Source: three-view drawing plus pictorial views. Frame: mm from the lowest corner of the part. Give positions to 0.01 mm unless a question says otherwise; leave off trailing zeros. Loops run counter-clockwise (first coordinate to the right, second up) from the corner with the lowest first, then second, coordinate; pieces in that order, holes last. Notation, with made-up numbers: (52, -6.75) -> (82, -6.75) arc R15 ccw to (82, 4.25) -> close; hole circle Ø2 at (-6, 58.5). An arc over 180 degrees is marked (long way). Put each result on its own line as item: value.
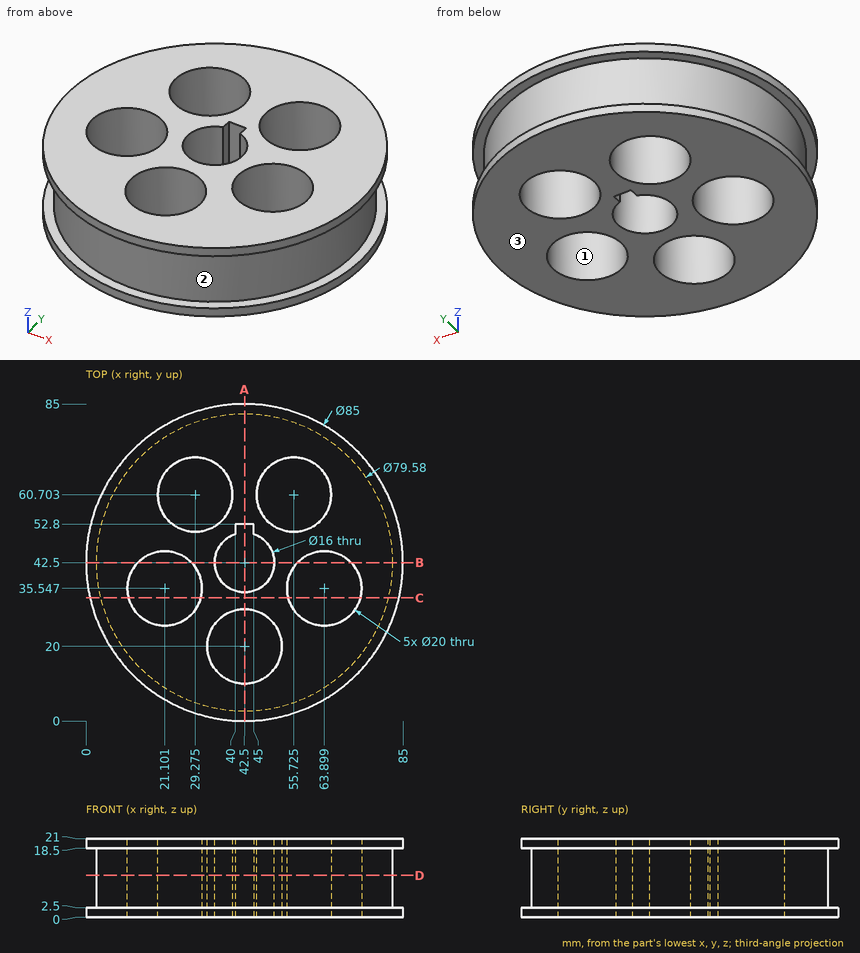
(1) Draft query along X for the marked faces 1, 2 and 3. Return one class per face: released by +X, released by -X, zero draft, split by the parting line, or undercut.
Calculated:
face 1: undercut
face 2: split by the parting line
face 3: zero draft
(2) Section C-C on y = 33. Return loops of the section in (x, z) (1 decimal).
Calculated:
outline: (1.1, 0) -> (11.4, 0) -> (11.4, 21) -> (1.1, 21) -> (1.1, 18.5) -> (3.9, 18.5) -> (3.9, 2.5) -> (1.1, 2.5) -> close; (30.8, 0) -> (54.2, 0) -> (54.2, 21) -> (30.8, 21) -> close; (73.6, 0) -> (83.9, 0) -> (83.9, 2.5) -> (81.1, 2.5) -> (81.1, 18.5) -> (83.9, 18.5) -> (83.9, 21) -> (73.6, 21) -> close
(3) First-contact query: P1, Ø1.4, axis at y = 51.5, z = 15, coming from the +X side (1 decimal); P2, Ø4, axis at y = 29, z = 6.5, coming from the +X side; P3, Ø1.5, axis at y = 56, z = 6.5, coming from the -X side. Flat tips, straight axial feed; report the tip coordinate or a pass-through.
Calculated:
P1: stops at x = 81.4
P2: stops at x = 80.59
P3: stops at x = 4.81
(4) Section D-D on z = 11.25. Return loops of the section in (x, y) (1 decimal).
Calculated:
outline: circle Ø79.6 at (42.5, 42.5); hole circle Ø20 at (21.1, 35.5); hole circle Ø20 at (29.3, 60.7); hole circle Ø20 at (42.5, 20); hole (40, 50.1) arc R8 ccw (long way) to (45, 50.1) -> (45, 52.8) -> (40, 52.8) -> close; hole circle Ø20 at (55.7, 60.7); hole circle Ø20 at (63.9, 35.5)
(5) Line query: probe 1 along Y at (x, z) = (42.5, 8.5); probe 2 along X at (y, z) = (38, 17.75) (1 decimal); probe 3 along X at (y, z) = (41, 6). Output: solid intervals per line, ascending. Write a range as from..to.
Calculated:
probe 1: y = 2.71..10, 30..34.5, 52.8..82.29
probe 2: x = 3..11.4, 30.8..35.9, 49.1..54.2, 73.6..82
probe 3: x = 2.74..12.72, 29.48..34.64, 50.36..55.52, 72.28..82.26
(6) Section A-A on x = 42.5. Return loops of the section in (y, z), then the cut area to 3 significant figures.
Calculated:
outline: (0, 0) -> (10, 0) -> (10, 21) -> (0, 21) -> (0, 18.5) -> (2.71, 18.5) -> (2.71, 2.5) -> (0, 2.5) -> close; (30, 0) -> (34.5, 0) -> (34.5, 21) -> (30, 21) -> close; (52.8, 0) -> (85, 0) -> (85, 2.5) -> (82.29, 2.5) -> (82.29, 18.5) -> (85, 18.5) -> (85, 21) -> (52.8, 21) -> close
area: 894 mm²
(7) Section B-B on y = 42.5. Return loops of the section in (x, z).
Calculated:
outline: (0, 0) -> (13.91, 0) -> (13.91, 21) -> (0, 21) -> (0, 18.5) -> (2.71, 18.5) -> (2.71, 2.5) -> (0, 2.5) -> close; (28.29, 0) -> (34.5, 0) -> (34.5, 21) -> (28.29, 21) -> close; (50.5, 0) -> (56.71, 0) -> (56.71, 21) -> (50.5, 21) -> close; (71.09, 0) -> (85, 0) -> (85, 2.5) -> (82.29, 2.5) -> (82.29, 18.5) -> (85, 18.5) -> (85, 21) -> (71.09, 21) -> close
